Here's how the part is built. I have some questions about the finished solid (model axes, mm). A direction names the side the tool comes from. Round coordinates to 2 decimals unless told otherwise and drop trailing zeros. Order: outer loops, then holes, each group sorted by start corner. A loop starts at its lowest first (then second) coordinate and runs counter-clockwise, first axis right, second up. Notation, with made-up numbers: (-18.75, 47.25) - (11.25, 47.25) arc R26 cw to (11.25, 77.25) - close; hole circle Ø6 at (1.25, -35.75). An arc over 180 degrees is marked (long way). One line per item, written item: value.
from build123d import *

# Parameters (mm, degrees)
F1_DEPTH = 10
F2_T     = 1
F3_W     = 12
F3_H     = 10
F4_DEPTH = 25
F5_W     = 236.8284271247
F5_H     = 11
F6_DEPTH = 1
F8_D     = 3.3


with BuildPart() as f1:
    # F0 (on Top) → F1 (new body)
    with BuildSketch(Plane.XY):
        Polygon((116, 0), (-116, 0), (-6, -110), (6, -110), align=None)
    extrude(amount=F1_DEPTH)

    # F2
    f2_openings = [f1.faces().sort_by_distance(p)[0] for p in [
        (0, -38.469945, 10),
    ]]
    offset(amount=F2_T, openings=f2_openings, kind=Kind.INTERSECTION)

    # F3 (on face) → F4 (cut)
    with BuildSketch(Plane(origin=(0, -110, 0), x_dir=(-1, 0, 0), z_dir=(0, 1, 0))):
        with Locations((0, 5)):
            Rectangle(F3_W, F3_H)
    extrude(amount=-F4_DEPTH, mode=Mode.SUBTRACT)

    # F5 (on face) → F6 (cut)
    with BuildSketch(Plane(origin=(0, 1, 0), x_dir=(-1, 0, 0), z_dir=(0, 1, 0))):
        with Locations((0, 4.5)):
            Rectangle(F5_W, F5_H)
    extrude(amount=-F6_DEPTH, mode=Mode.SUBTRACT)

    # F8 (through all)
    with Locations(Plane.XY):
        with Locations((0, -41), (0, -61)):
            Hole(F8_D / 2)


solid = f1.part
Q1. Which directions (+Z, -Z, +X, -X, +Y, -Y) give clear straight access to the entire face, cutting with the end or side of a thin tool? Please do faces 5 (the flat face through (-62, -54, 5)), 6 (the flat face through (0, -111, -0.4)).
Results list:
face 5: +Z, +Y
face 6: +Z, -Z, +X, -X, -Y
Q2. We'd pull the mould along X, two halves only. Please class faces 1 (the flat face through (-2, -42, 0)), 2 (the flat face through (-62.691, -54.723, 4.423)), 3 (the flat face through (61.137, -56.277, 4.423)), 4 (the flat face through (0.5, 0, -0.4)): released by +X, released by -X, zero draft, split by the parting line, or undercut.
Results list:
face 1: undercut
face 2: released by -X
face 3: released by +X
face 4: zero draft
Q3. Will these pins go through, and if not, where does the flat tip stop? pin 1 (5 mm diameter, centred on x = 19.5, y = -26.5, fed in from +Z); pin 2 (0.8 mm diameter, centred on y = -110.5, z = 6.5, fed in from +X); pin 3 (3 mm diameter, centred on x = 51.5, z = 8.5, fed in from +Y); pin 4 (2.5 mm diameter, centred on x = 0, y = -61, fed in from +Z).
Results list:
pin 1: z = 0
pin 2: x = 7.31
pin 3: y = -63
pin 4: through
Q4. If we section it at B-B, the plane y = -76: Please give me the cut outline in (x, z).
Results list:
outline: (-41.41, -1) - (41.41, -1) - (41.41, 10) - (40, 10) - (40, 0) - (-40, 0) - (-40, 10) - (-41.41, 10) - close
Q5. If we section it at A-A, the plane z = 6: Please give me the cut outline in (x, y), then the cut area to 3 significant figures.
Results list:
outline: (-117.41, 0) - (-6.41, -111) - (-6, -111) - (-6, -110) - (-116, 0) - close; (6, -111) - (6.41, -111) - (117.41, 0) - (116, 0) - (6, -110) - close
area: 313 mm²
Q6. If I drill on line 1 along Y through (x, z) = (0, -0.5); line 2 along Z through (x, y) = (34.5, -60.5); line 3 along X through (y, z) = (-98.5, 8), over which ranges is the centre line in solid material (lowest first)?
Results list:
line 1: -111 to -62.65, -59.35 to -42.65, -39.35 to 0
line 2: -1 to 0
line 3: -18.91 to -17.5, 17.5 to 18.91
Q7. If we section it at D-D, the plane x = 83: Please give me the cut outline in (y, z), then the cut area to 3 significant figures.
Results list:
outline: (-34.41, -1) - (0, -1) - (0, 0) - (-33, 0) - (-33, 10) - (-34.41, 10) - close
area: 48.6 mm²
Q8. If we section it at C-C, the plane x = 24: Please give me the cut outline in (y, z).
Results list:
outline: (-93.41, -1) - (0, -1) - (0, 0) - (-92, 0) - (-92, 10) - (-93.41, 10) - close
